Part model, mm, in its own coordinate system. A direction names the side the tool comes from. Coordinates: 2 decimals unless noted, no trailing zeros. Order: outer loops, then holes, each group sorted by start corner. A loop starts at its lowest first (then second) coordinate and runs counter-clockwise, first axis right, second up.
1) Cut at C-C (y = -1.2). List the corners of the cut face in (x, z), and give its area (3 significant figures).
2) Pin check, flat tips, straight feed: pin 1 Ø5.5 at (x, z) = (-44, 6.5) entering from -Y; pin 2 Ø0.8 at (x, y) = (-29, -1) entering from -Z; pin 3 Ø0.8 at (x, y) = (31.5, -1) entering from +Z; pin 4 Ø0.6 at (y, z) = (-0.5, -1) entering from -X. Stop position of each tip, or through.
3) Wall check: L1, parallel to X at y = -0.95, z = 6.5; L2, parallel to X at y = -0.75, z = 26.5; L3, parallel to Z at x = -9.5, y = -0.6. Give the ranges that are in metal, low to high.
4) Tool access for faces 1 (the cylindrical face through (-73.57, -0.74, 50)), 2 (the cylindrical face through (-73.5, -0.74, -50.07)), 3 (the cylindrical face through (73.57, -0.74, -50)), 4 (the cylindrical face through (73.5, -0.74, 50.07)): list every direction of +Z, -Z, +X, -X, +Y, -Y with a clear straight run to the whole face (end or side of a thin tool).
5) Cut at A-A (z = 33). List the corners of the cut face in (x, y), and give its area (3 significant figures).
6) Mould opens along X. For faces 5 (the cylindrical face through (74.5, 0.25, -51.07)), 6 (the cylindrical face through (-40.53, -0.49, 16.04)), 7 (the cylindrical face through (-74.57, 0.25, -51)), 8 (the cylindrical face through (-40.53, -0.49, 6.04)) say: +X half, -X half, draft (parallel to the pull), parting line (faces both ways), or undercut.
7) Cut at D-D (x = 3). List the corners of the cut face in (y, z).
8) Cut at B-B (z = 16.5). List the corners of the cut face in (x, y).
```python
from build123d import *

# Parameters (mm, degrees)
EXTRUDE_5_DEPTH      = 0.5
EXTRUDE_6_DEPTH      = 1.5
SKETCH_19_W          = 55
SKETCH_19_H          = 75
CUT_EXTRUDE_10_DEPTH = 33
SKETCH_20_W          = 10
SKETCH_20_H          = 7
CUT_EXTRUDE_11_DEPTH = 33
SKETCH_21_R          = 3.5
CUT_EXTRUDE_12_DEPTH = 33


with BuildPart() as part:
    # 草图16 → 凸台-拉伸5 (new body)
    with BuildSketch(Plane(origin=(0, 0, 0), x_dir=(1, 0, 0), z_dir=(0, 1, 0))):
        with BuildLine():
            Line((71, -52.5), (-71, -52.5))
            ThreePointArc((-71, -52.5), (-74.535533906, -51.035533906), (-76, -47.5))
            Line((-76, -47.5), (-76, 47.5))
            ThreePointArc((-76, 47.5), (-74.535533906, 51.035533906), (-71, 52.5))
            Line((-71, 52.5), (71, 52.5))
            ThreePointArc((71, 52.5), (74.535533906, 51.035533906), (76, 47.5))
            Line((76, 47.5), (76, -47.5))
            ThreePointArc((76, -47.5), (74.535533906, -51.035533906), (71, -52.5))
        make_face()
    extrude(amount=EXTRUDE_5_DEPTH)

    # 草图18 → 凸台-拉伸6 (add)
    with BuildSketch(Plane.XZ):
        with BuildLine():
            Line((70, -51.5), (-70, -51.5))
            ThreePointArc((-70, -51.5), (-73.535533906, -50.035533906), (-75, -46.5))
            Line((-75, -46.5), (-75, 46.5))
            ThreePointArc((-75, 46.5), (-73.535533906, 50.035533906), (-70, 51.5))
            Line((-70, 51.5), (70, 51.5))
            ThreePointArc((70, 51.5), (73.535533906, 50.035533906), (75, 46.5))
            Line((75, 46.5), (75, -46.5))
            ThreePointArc((75, -46.5), (73.535533906, -50.035533906), (70, -51.5))
        make_face()
    extrude(amount=EXTRUDE_6_DEPTH)

    # 草图19 → 切除-拉伸10 (cut)
    with BuildSketch(Plane(origin=(0, 0.5, 0), x_dir=(1, 0, 0), z_dir=(0, 1, 0))):
        with Locations((-6.5, -1)):
            Rectangle(SKETCH_19_W, SKETCH_19_H)
    extrude(amount=-CUT_EXTRUDE_10_DEPTH, mode=Mode.SUBTRACT)

    # 草图20 → 切除-拉伸11 (cut)
    with BuildSketch(Plane(origin=(0, 0.5, 0), x_dir=(1, 0, 0), z_dir=(0, 1, 0))):
        with Locations((33, -24)):
            Rectangle(SKETCH_20_W, SKETCH_20_H)
    extrude(amount=-CUT_EXTRUDE_11_DEPTH, mode=Mode.SUBTRACT)

    # 草图21 → 切除-拉伸12 (cut)
    with BuildSketch(Plane(origin=(0, 0.5, 0), x_dir=(1, 0, 0), z_dir=(0, 1, 0))):
        with Locations(Location((-44, -6.5, 0), (0, 0, 270))):
            Circle(SKETCH_21_R)
        with Locations(Location((-44, -16.5, 0), (0, 0, 270))):
            Circle(SKETCH_21_R)
        with Locations(Location((-44, -26.5, 0), (0, 0, 270))):
            Circle(SKETCH_21_R)
    extrude(amount=-CUT_EXTRUDE_12_DEPTH, mode=Mode.SUBTRACT)


solid = part.part
```
Geometry check:
1. outline: (-75, -46.5) arc R5 ccw to (-70, -51.5) - (70, -51.5) arc R5 ccw to (75, -46.5) - (75, 46.5) arc R5 ccw to (70, 51.5) - (-70, 51.5) arc R5 ccw to (-75, 46.5) - close; hole circle Ø7 at (-44, 6.5); hole circle Ø7 at (-44, 16.5); hole circle Ø7 at (-44, 26.5); hole (-34, -36.5) - (21, -36.5) - (21, 38.5) - (-34, 38.5) - close; hole (28, 20.5) - (38, 20.5) - (38, 27.5) - (28, 27.5) - close
1. area: 11,100 mm2
2. pin 1: passes through
2. pin 2: stops at z = -51.5
2. pin 3: stops at z = 51.5
2. pin 4: stops at x = -75
3. L1: x = -75 to -47.5, -40.5 to -34, 21 to 75
3. L2: x = -75 to -47.5, -40.5 to -34, 21 to 28, 38 to 75
3. L3: z = -51.5 to -36.5, 38.5 to 51.5
4. face 1: +Z, -X, -Y
4. face 2: -Z, -X, -Y
4. face 3: -Z, +X, -Y
4. face 4: +Z, +X, -Y
5. outline: (-76, 0) - (-75, 0) - (-75, -1.5) - (-34, -1.5) - (-34, 0.5) - (-76, 0.5) - close; (21, -1.5) - (75, -1.5) - (75, 0) - (76, 0) - (76, 0.5) - (21, 0.5) - close
5. area: 191 mm2
6. face 5: +X half
6. face 6: undercut
6. face 7: -X half
6. face 8: undercut
7. outline: (-1.5, -51.5) - (0, -51.5) - (0, -52.5) - (0.5, -52.5) - (0.5, -36.5) - (-1.5, -36.5) - close; (-1.5, 38.5) - (0.5, 38.5) - (0.5, 52.5) - (0, 52.5) - (0, 51.5) - (-1.5, 51.5) - close
8. outline: (-76, 0) - (-75, 0) - (-75, -1.5) - (-47.5, -1.5) - (-47.5, 0.5) - (-76, 0.5) - close; (-40.5, -1.5) - (-34, -1.5) - (-34, 0.5) - (-40.5, 0.5) - close; (21, -1.5) - (75, -1.5) - (75, 0) - (76, 0) - (76, 0.5) - (21, 0.5) - close
